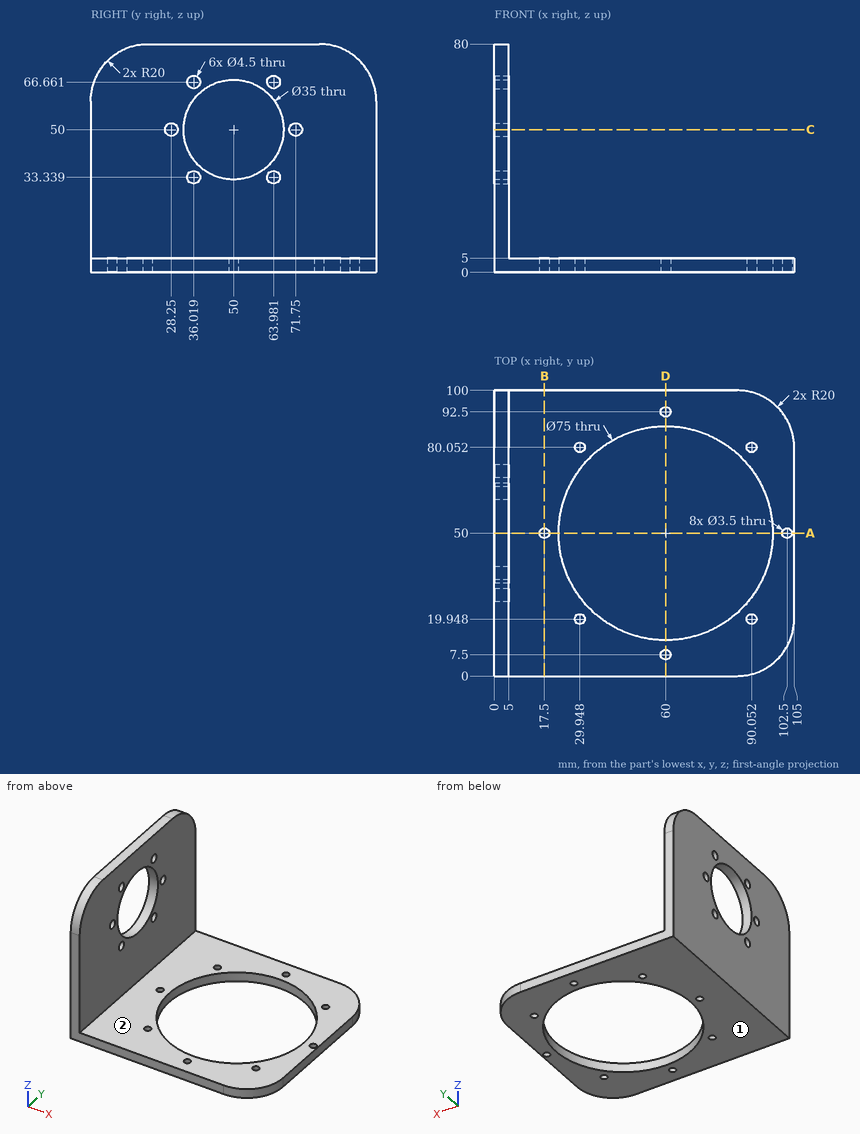
Part print with two shaded views. Sizes in mm from the minimum x, y, z corner. A direction names the side the tool comes from. Round coordinates to 2 decimals unless told otherwise and drop trailing zeros. Order: outer loops, then holes, each group sorted by start corner. A loop starts at its lowest first (then second) coordinate and runs counter-clockwise, first axis right, second up. Notation, with made-up numbers: M 47,82.25 L 57,82.25 A23 cw 57,96.25 Z; hole C 73.5,81.25 d1. An arc over 180 degrees is marked long. Answer in a Markdown table with one row per item. Add a question column.
Q1. Pin check, flat tips, straight feed: pin 1 (1 mm diameter, centred on y = 72.5, z = 36, fed in from +X); pin 2 (2.5 mm diameter, centred on y = 36.02, z = 66.66, fed in from +X); pin 3 (5 mm diameter, centred on x = 59.5, y = 11.5, fed in from +Z). Stop position of each tip, or through.
Q2. Cut at C-C on z = 50. Give the cut face in (x, y).
Q3. Cut at B-B on x = 17.5. Give the cut face in (y, z).
Q4. Wall check: L1, parallel to X at y = 50, z = 3.8; L2, parallel to Z at x = 14.5, y = 49; L3, parallel to X at y = 27, z = 4.5. Give the ranges that are in metal, low to high. Write a range as from..to.
Q5. Cut at A-A on y = 50. Give the cut face in (x, z).
Q6. 3-axis set-ups, long thin cutter, end or side, ignore diameter. For the marked faces 1 and 2: which of +Z, -Z, +X, -X, +Y, -Y reach the whole face in a straight line?
Q7. Cut at D-D on x = 60. Give the cut face in (y, z).
Established:
| question | item | result |
|---|---|---|
| 1 | pin 1 | stops at x = 5 |
| 1 | pin 2 | passes through |
| 1 | pin 3 | stops at z = 5 |
| 2 | outline | M 0,0 L 5,0 L 5,26 L 0,26 Z; M 0,30.5 L 5,30.5 L 5,32.5 L 0,32.5 Z; M 0,67.5 L 5,67.5 L 5,69.5 L 0,69.5 Z; M 0,74 L 5,74 L 5,100 L 0,100 Z |
| 3 | outline | M 0,0 L 48.25,0 L 48.25,5 L 0,5 Z; M 51.75,0 L 100,0 L 100,5 L 51.75,5 Z |
| 4 | L1 | x = 0..15.75, 19.25..22.5, 97.5..100.75, 104.25..105 |
| 4 | L2 | z = 0..5 |
| 4 | L3 | x = 0..30.38, 89.62..105 |
| 5 | outline | M 0,0 L 15.75,0 L 15.75,5 L 5,5 L 5,32.5 L 0,32.5 Z; M 0,67.5 L 5,67.5 L 5,80 L 0,80 Z; M 19.25,0 L 22.5,0 L 22.5,5 L 19.25,5 Z; M 97.5,0 L 100.75,0 L 100.75,5 L 97.5,5 Z; M 104.25,0 L 105,0 L 105,5 L 104.25,5 Z |
| 6 | face 1 | -Z, +X, -X, +Y, -Y |
| 6 | face 2 | +Z, +X, +Y, -Y |
| 7 | outline | M 0,0 L 5.75,0 L 5.75,5 L 0,5 Z; M 9.25,0 L 12.5,0 L 12.5,5 L 9.25,5 Z; M 87.5,0 L 90.75,0 L 90.75,5 L 87.5,5 Z; M 94.25,0 L 100,0 L 100,5 L 94.25,5 Z |
